Check sheet for the modelled part. Datum: model origin and axes. Units: mm. Coordinates: 2 decimals unless noted, no trailing zeros. Write each loop counter-clockwise with the first axis right and the second up, starting at its lowest first coordinate (ties: lowest second). Pieces come first, ordered by that corner, then holes. Notation, with made-up numbers: (76.5, 66.5) - (105.5, 66.5) arc R23 ccw to (105.5, 97.5) - close; hole circle Ø1 at (-25.5, 18.25). An arc over 180 degrees is marked (long way). Answer as CSV lines item,"result". Start each with the question number.
from build123d import *

# Parameters (mm, degrees)
SKETCH_R      = 2.5
EXTRUDE_DEPTH = 5


with BuildPart() as part:
    # Sketch → Extrude (new body)
    with BuildSketch(Plane.XY):
        with BuildLine():
            ThreePointArc((0, 5), (-5, 0), (0, -5))
            Line((100, -5), (0, -5))
            ThreePointArc((100, -5), (105, 0), (100, 5))
            Line((0, 5), (100, 5))
        make_face()
        Circle(SKETCH_R, mode=Mode.SUBTRACT)
        with Locations((100, 0)):
            Circle(SKETCH_R, mode=Mode.SUBTRACT)
    extrude(amount=EXTRUDE_DEPTH)


with BuildPart() as part_1:
    # Extrude placement: moved
    add(part.part.moved(Location((68.762068, 37.732329, -2.433251))))


solid = part_1.part
(1) Material ranges on probe 1 along X at (y, z) = (37.75, 0.7); probe 2 along X at (y, z) = (38, -1.4); probe 3 along Y at (x, z) = (68.5, -1.25), recorded low to high. Write a range as from..to.
(2) Cross-section at B-B on y = 41.25. Record the boundary of the cut face in (x, z), plus the area to 3 significant figures.
(3) Cross-section at A-A on z = 0.9. Record the boundary of the cut face in (x, y).
Checked values:
1,probe 1,"63.76..66.26, 71.26..166.26, 171.26..173.76"
1,probe 2,"63.77..66.28, 71.25..166.28, 171.25..173.75"
1,probe 3,"32.74..35.25, 40.22..42.73"
2,outline,"(65.21, -2.43) - (172.32, -2.43) - (172.32, 2.57) - (65.21, 2.57) - close"
2,area,"536 mm^2"
3,outline,"(68.76, 32.73) - (168.76, 32.73) arc R5 ccw to (168.76, 42.73) - (68.76, 42.73) arc R5 ccw to start; hole circle Ø5 at (68.76, 37.73); hole circle Ø5 at (168.76, 37.73)"
